Verification items for the finished model (mm, model axes). Face numbers are marked on the shaded views. A direction names the side the tool comes from. Give positions to 0.01 mm unless a question says otherwise; leave off trailing zeros. Loops run counter-clockwise (first coordinate to the right, second up) from the corner with the lowest first, then second, coordinate; pieces in that order, holes last. Notation, with made-up numbers: M 65,28 L 72,28 A26 ccw 72,52 Z; hole C 43.25,83 d4. An arc over 180 degrees is marked long. Put each result on its own line as item: value. Start each with the question number.
Autodesk Inventor part; units mm, degrees
ref_plane "YZ Plane" through (0, 0, 0) normal (1, 0, 0) x (0, 1, 0)
ref_plane "XZ Plane" through (0, 0, 0) normal (0, 1, 0) x (-1, 0, 0)
ref_plane "XY Plane" through (0, 0, 0) normal (0, 0, 1) x (1, 0, 0)
sketch "Sketch1" plane through (0, 0, 0) normal (0, 0, 1) x (1, 0, 0)
  circle A0 centre (0, 0) radius 45
  line L0 (0, -45) -> (500, -45)
  line L1 (500, -45) -> (500, -25)
  line L2 (500, -25) -> (0, -25)
  line L3 (0, -25) -> (0, -45)
  line L4 (0, 45) -> (600, 45)
  line L5 (600, 45) -> (600, 25)
  line L6 (600, 25) -> (0, 25)
  line L7 (0, 25) -> (0, 45)
  circle A1 centre (0, 0) radius 25
  point P0 (0, -25)
  point P1 (0, 25)
  dimension "d0" = 90
  dimension "d1" = 20
  dimension "d2" = 20
  dimension "d4" = 500
  dimension "d9" = 600
extrude "Extrusion1" add sketch "Sketch1" along normal blind 49 contours L7 A1 L3 A0 | L4 L5 L6 A0 | A0 L6 L7 | L3 L2 A0 | A0 L2 L1 L0
properties part number "J15BF.1.40_Xaxis_B"
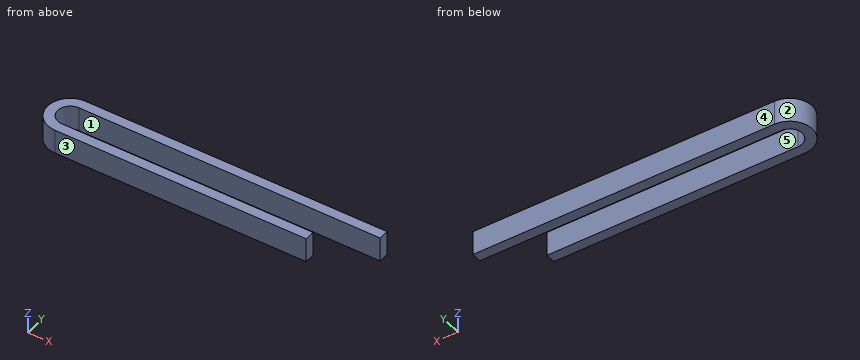
Q1. Release check for a two-part mould opening along Y. For the marked faces 3, 4 and 5 record: pulls with the +Y half, pulls with the -Y half, needs draft (parallel to the pull), parting line crosses it, or undercut.
Q2. Go/stop test with flat-tipped pins: pin 1 (1 mm diameter, centred on y = 10.5, z = 22, fed in from +X); pin 2 (10 mm diameter, centred on y = -36.5, z = 31.5, fed in from +X); pin 3 (2 mm diameter, centred on y = -28.5, z = 36.5, fed in from -X). Record where each tip stops, or that it passes through.
Q3. Cross-section at A-A, the plane x = 71. Record the boundary of the cut face in (y, z), then the cut area to 3 significant figures.
Q4. Cross-section at C-C, the plane y = 36. Record the boundary of the cut face in (x, z).
Q5. Cross-section at D-D, the plane x = 515. Record the boundary of the cut face in (y, z).
Q6. Set-up check for the marked faces 1 and 2: record each of +Z, -Z, +X, -X, +Y, -Y from which the full face is reachable in a straight line by a thin tool's end or side.
Q7. Cross-section at B-B, the plane z = 11. Record the boundary of the cut face in (x, y), then the cut area to 3 significant figures.
Q8. Scan lines: L1, parallel to Y at x = 353, z = 15.5; L2, parallel to Y at x = 568.5, z = 42; L3, parallel to Y at x = -2, z = 24.5. Record each from-to range of solid material in increasing order.
Ans:
1. face 3: pulls with the -Y half
1. face 4: pulls with the +Y half
1. face 5: undercut
2. pin 1: stops at x = -22.45
2. pin 2: stops at x = 500
2. pin 3: stops at x = -35.62
3. outline: M -45,0 L -25,0 L -25,49 L -45,49 Z; M 25,0 L 45,0 L 45,49 L 25,49 Z
3. area: 1,960 mm^2
4. outline: M -27,0 L 600,0 L 600,49 L -27,49 Z
5. outline: M 25,0 L 45,0 L 45,49 L 25,49 Z
6. face 1: +Z, -Z, +X
6. face 2: +Z, -Z, -X
7. outline: M 0,-45 L 500,-45 L 500,-25 L 0,-25 A25 cw 0,25 L 600,25 L 600,45 L 0,45 A45 ccw Z
7. area: 24,200 mm^2
8. L1: y = -45 to -25, 25 to 45
8. L2: y = 25 to 45
8. L3: y = -44.96 to -24.92, 24.92 to 44.96
